Autodesk Inventor part; units mm, degrees
ref_plane "YZ Plane" through (0, 0, 0) normal (1, 0, 0) x (0, 1, 0)
ref_plane "XZ Plane" through (0, 0, 0) normal (0, 1, 0) x (-1, 0, 0)
ref_plane "XY Plane" through (0, 0, 0) normal (0, 0, 1) x (1, 0, 0)
sketch "Sketch1" plane through (0, 0, 0) normal (0, 0, 1) x (1, 0, 0)
  circle A0 centre (0, 0) radius 19.05
  circle A1 centre (0, 0) radius 5.6063
  dimension "d0" = 11.2125
  dimension "d2" = 38.1
extrude "Extrusion1" add sketch "Sketch1" along normal blind 5
sketch "Sketch2" plane through (0, 0, 5) normal (0, 0, 1) x (1, 0, 0)
  circle A0 centre (0, 0) radius 5.6063
  circle A1 centre (0, 0) radius 19.05
  circle A2 centre (0, 0) radius 14.2875
  circle A3 centre (0, 0) radius 11.1125
  dimension "d5" = 28.575
  dimension "d26" = 22.225
extrude "Extrusion2" add sketch "Sketch2" along normal blind 30 contours A3
sketch "Sketch3" plane through (0, 0, 5) normal (0, 0, 1) x (1, 0, 0)
  circle A0 centre (0, 0) radius 11.1125
  circle A1 centre (0, 14.2875) radius 1.75
  dimension "d11" = 14.2875
  dimension "d12" = 3.5
extrude "Extrusion3" cut sketch "Sketch3" against normal through all contours A1
sketch "Sketch4" plane through (0, 0, 0) normal (1, 0, 0) x (0, 1, 0)
  line L0 (11.1125, 35) -> (11.1125, 5)
  line L1 (11.1125, 5) -> (12.5375, 5)
  line L2 (12.5375, 5) -> (12.5375, 0)
  line L3 (12.5375, 0) -> (5.6063, 0)
  line L4 (5.6063, 0) -> (5.6063, 35)
  line L5 (5.6063, 35) -> (11.1125, 35)
  line L6 (-19.05, 0) -> (-19.05, 5)
  line L7 (-19.05, 5) -> (-11.1125, 5)
  line L8 (-11.1125, 5) -> (-11.1125, 35)
  line L9 (-11.1125, 35) -> (-5.6063, 35)
  line L10 (-5.6063, 35) -> (-5.6063, 0)
  line L11 (-5.6063, 0) -> (-19.05, 0)
  line L12 (19.05, 5) -> (19.05, 0)
  line L13 (19.05, 0) -> (16.0375, 0)
  line L14 (16.0375, 0) -> (16.0375, 5)
  line L15 (16.0375, 5) -> (19.05, 5)
  line L16 (-19.05, 5) -> (-11.1125, 5)
  line L17 (-11.1125, 35) -> (-19.05, 5)
  line L18 (-11.1125, 35) -> (-11.1125, 5)
  point P0 (0, 0)
extrude "Extrusion4" add sketch "Sketch4" along normal mid plane 5 contours L17 L8 L7
sketch "Sketch5" plane through (0, 0, 35) normal (0, 0, 1) x (1, 0, 0)
  circle A0 centre (0, 0) radius 11.1125
  line L0 (2.5, -19.05) -> (0, -19.05)
  line L1 (2.5, -11.1125) -> (2.5, -19.05)
  line L2 (0, -11.1125) -> (2.5, -11.1125)
  line L3 (-2.5, -11.1125) -> (0, -11.1125)
  line L4 (-2.5, -19.05) -> (-2.5, -11.1125)
  line L5 (0, -19.05) -> (-2.5, -19.05)
  line L6 (-2.5, -11.1125) -> (2.5, -11.1125)
  line L7 (2.5, -11.1125) -> (2.5, -10.8276)
  line L8 (2.5, -10.8276) -> (-2.5, -10.8276)
  line L9 (-2.5, -10.8276) -> (-2.5, -11.1125)
extrude "Extrusion5" add sketch "Sketch5" against normal up to surface (30 mm away) contours L8 A0 | A0 L3 L9 | L7 L2 A0 picked at (-0.5582, -10.8803)
sketch "Sketch6" plane through (0, 0, 0) normal (0, 0, -1) x (-1, 0, 0)
  circle A0 centre (0, 0) radius 19.05
  circle A1 centre (0, 0) radius 25.4
  dimension "d19" = 6.35
extrude "Extrusion6" cut sketch "Sketch6" against normal through all
pattern_circular "Circular Pattern1" count 3 over 360 about axis through (0, 0, 5) along (0, 0, 1) of "Extrusion6", "Extrusion5", "Extrusion4", "Extrusion3"
properties part number "GUIDE"
Could you check a few things on this model? Use its own coordinates, in mm. A direction names the side the tool comes from. Round coordinates to 2 decimals unless told otherwise and drop trailing zeros. Write each loop counter-clockwise with the first axis right and the second up, starting at its lowest first coordinate (ties: lowest second). Pieces come first, ordered by that corner, then holes. Notation, with made-up numbers: M -0.5,59 L 38.5,59 A12 ccw 38.5,68 Z; hole C 65.5,8.25 d1. An arc over 180 degrees is marked long. Write each question's results on one line, items separated by ' | '. Start each with the question number.
1. Imagine slicing it at A-A on x = 0. List the corners of the cut face in (y, z) for me.
2. Imagine slicing it at C-C on z = 8. List the corners of the cut face in (x, y) for me (1 decimal).
3. I'm going to push flat-ended pins straight in: pin 1 Ø12 at (y, z) = (-4.5, 29) entering from -X; pin 2 Ø3 at (x, y) = (0, 14.29) entering from -Z; pin 3 Ø4 at (x, y) = (12.37, -7.14) entering from +Z; pin 4 Ø4 at (y, z) = (-13, 17.5) entering from +X. Where does each tip first touch, or does it pass through?
4. I need wall thicknesses on L1, parallel to X at y = -7, z = 4; L2, parallel to Z at x = -9.5, y = -6; L3, parallel to X at y = 5, z = 21. Which ranges of each line are inside material? Lowest first, please. Write a range as from..to.
5. Imagine slicing it at B-B on y = 0. List the corners of the cut face in (x, z) for me, and give its area (3 significant figures).
6. Thinking about a two-plate mould opening in X: for faces 1 (the face through (-0.38, 12.58, 2.54)), 2 (the face through (13.181, -8.696, 2.535)), 3 (the face through (-2.5, -14, 17)), 4 (the face through (-5, 3, 35)), which applies, +X half, -X half, draft (parallel to the pull), parting line (faces both ways), or undercut?
7. On a 3-axis mill with a long thin cutter (end or side, diameter ignored), from which of +Z, -Z, +X, -X, +Y, -Y can I reach the whole of each face in a straight line? I mean faces 5 (the face through (-9.559, -5.666, 19.79)), 6 (the face through (-0.13, 11.11, 19.79)), 7 (the face through (2.5, -14, 17)). Say none if no direction works.
8. Imagine slicing it at D-D on x = 12.5. List the corners of the cut face in (y, z) for me, and give its area (3 significant figures).
Result sheet:
1) outline: M -19.05,0 L -5.61,0 L -5.61,35 L -11.11,35 L -19.05,5 Z; M 5.61,0 L 12.54,0 L 12.54,5 L 11.11,5 L 11.11,35 L 5.61,35 Z; M 16.04,0 L 19.05,0 L 19.05,5 L 16.04,5 Z
2) outline: M -17.1,7 L -10.6,3.2 A11.1 ccw -2.5,-10.8 L -2.5,-18.3 L 2.5,-18.3 L 2.5,-10.8 A11.1 ccw 10.6,3.2 L 17.1,7 L 14.6,11.3 L 8.1,7.6 A11.1 ccw -8.1,7.6 L -14.6,11.3 Z; hole C 0,0 d11.2
3) pin 1: stops at x = -11.11 | pin 2: passes through | pin 3: stops at z = 5 | pin 4: stops at x = 2.5
4) L1: x = -17.72..-14.12, -10.63..10.63, 14.12..17.72 | L2: z = 0..5 | L3: x = -13.66..-2.54, 2.54..13.66
5) outline: M -19.05,0 L -5.61,0 L -5.61,35 L -11.11,35 L -11.11,5 L -19.05,5 Z; M 5.61,0 L 19.05,0 L 19.05,5 L 11.11,5 L 11.11,35 L 5.61,35 Z | area: 465 mm^2
6) face 1: undercut | face 2: undercut | face 3: -X half | face 4: draft
7) face 5: +Z, -X | face 6: +Z, +Y | face 7: +Z, +X, -Y
8) outline: M -14.38,0 L -8.89,0 L -8.89,5 L -14.38,5 Z; M -5.4,0 L 14.38,0 L 14.38,5 L 10.1,5 L 10.1,16.99 L 4.33,27.9 L 4.33,5 L -5.4,5 Z | area: 227 mm^2
